```python
from build123d import *

# Parameters (mm, degrees)
F1_DEPTH = 15
F2_W     = 8.1
F2_H     = 8.1
F3_DEPTH = 15.001


with BuildPart() as f1:
    # F0 (on Top) → F1 (new body)
    with BuildSketch(Plane.XY):
        Polygon((9.68382, -9.550715), (10.192379, -9.560642), (10.750372, -9.002649), (11.202993, -8.356238), (11.104907, -7.857129), (10.443332, -6.402182), (9.825447, -5.605176), (9.499566, -5.342395), (8.382424, -4.808387), (7.960216, -4.101107), (8.739034, -1.961321), (9.517096, -1.690903), (10.716129, -1.999914), (11.134681, -2.008084), (12.120314, -1.794712), (13.562332, -1.105409), (13.958292, -0.786118), (14.027068, 0), (13.958292, 0.786118), (13.562332, 1.105409), (12.120314, 1.794712), (11.134681, 2.008084), (10.716129, 1.999914), (9.517096, 1.690903), (8.739034, 1.961321), (7.960216, 4.101107), (8.382424, 4.808387), (9.499566, 5.342395), (9.825447, 5.605176), (10.443332, 6.402182), (11.104907, 7.857129), (11.202993, 8.356238), (10.750372, 9.002649), (10.192379, 9.560642), (9.68382, 9.550715), (8.136095, 9.15184), (7.243903, 8.68174), (6.928526, 8.406442), (6.208641, 7.399001), (5.43879, 7.106025), (3.466753, 8.244581), (3.335552, 9.05778), (3.848079, 10.184939), (3.928805, 10.595713), (3.889828, 11.603424), (3.461401, 13.14323), (3.215719, 13.588618), (2.453486, 13.792858), (1.667367, 13.861634), (1.28417, 13.527134), (0.354935, 12.22672), (-0.026349, 11.293113), (-0.090983, 10.879501), (0.005123, 9.645024), (-0.396296, 8.925741), (-2.638814, 8.530325), (-3.262033, 9.068937), (-3.593939, 10.261836), (-3.796139, 10.628398), (-4.473741, 11.375294), (-5.791704, 12.279467), (-6.266198, 12.462733), (-6.981384, 12.129236), (-7.627795, 11.676614), (-7.706329, 11.174057), (-7.582274, 9.580582), (-7.274243, 8.620313), (-7.057892, 8.261922), (-6.190763, 7.378034), (-6.035921, 6.569004), (-7.499621, 4.824634), (-8.323248, 4.836637), (-9.344283, 5.537106), (-9.734799, 5.687937), (-10.733969, 5.824539), (-12.324777, 5.670005), (-12.806062, 5.505396), (-13.139559, 4.790209), (-13.343798, 4.027977), (-13.080922, 3.592515), (-11.961624, 2.451584), (-11.10841, 1.913973), (-10.712305, 1.778497), (-9.479894, 1.658779), (-8.841244, 1.138556), (-8.841244, -1.138556), (-9.479894, -1.658779), (-10.712305, -1.778497), (-11.10841, -1.913973), (-11.961624, -2.451584), (-13.080922, -3.592515), (-13.343798, -4.027977), (-13.139559, -4.790209), (-12.806062, -5.505396), (-12.324777, -5.670005), (-10.733969, -5.824539), (-9.734799, -5.687937), (-9.344283, -5.537106), (-8.323248, -4.836637), (-7.499621, -4.824634), (-6.035921, -6.569004), (-6.190763, -7.378034), (-7.057892, -8.261922), (-7.274243, -8.620313), (-7.582274, -9.580582), (-7.706329, -11.174057), (-7.627795, -11.676614), (-6.981384, -12.129236), (-6.266198, -12.462733), (-5.791704, -12.279467), (-4.473741, -11.375294), (-3.796139, -10.628398), (-3.593939, -10.261836), (-3.262033, -9.068937), (-2.638814, -8.530325), (-0.396296, -8.925741), (0.005123, -9.645024), (-0.090983, -10.879501), (-0.026349, -11.293113), (0.354935, -12.22672), (1.28417, -13.527134), (1.667367, -13.861634), (2.453486, -13.792858), (3.215719, -13.588618), (3.461401, -13.14323), (3.889828, -11.603424), (3.928805, -10.595713), (3.848079, -10.184939), (3.335552, -9.05778), (3.466753, -8.244581), (5.43879, -7.106025), (6.208641, -7.399001), (6.928526, -8.406442), (7.243903, -8.68174), (8.136095, -9.15184), align=None)
    extrude(amount=F1_DEPTH)

    # F2 (on face) → F3 (cut, through all)
    with BuildSketch(Plane.XY.offset(15)):
        Rectangle(F2_W, F2_H)
    extrude(amount=-F3_DEPTH, mode=Mode.SUBTRACT)


solid = f1.part
```
Check sheet for the modelled part. Datum: model origin and axes. Units: mm. A direction names the side the tool comes from. Coordinates: 2 decimals unless noted, no trailing zeros. Order: outer loops, then holes, each group sorted by start corner. A loop starts at its lowest first (then second) coordinate and runs counter-clockwise, first axis right, second up. Notation, with made-up numbers: M 22.5,-8 L 26.5,-8 A25 cw 26.5,9 Z; hole C 13,-35.75 d9. An arc over 180 degrees is marked long. Write each question's results on one line, items separated by ' | '. Start each with the question number.
1. Mould release check, pull along Y, two halves, no side actions. Record for faces 6 (the face through (0, -6, 0)), 7 (the face through (-12.5, -3, 7.4)), 8 (the face through (-8.827, 5.182, 7.395)): +Y half, -Y half, draft (parallel to the pull), parting line (faces both ways), or undercut.
2. Material ranges on probe 1 along Y at (x, z) = (9.75, 6); probe 2 along Y at (x, z) = (-7, 9.25); probe 3 along Y at (x, z) = (-1.75, 11.5), recorded low to high.
3. Go/stop test with flat-tipped pins: P1, Ø2.5, axis at y = 1.5, z = 8, coming from the +X side; P2, Ø8, axis at x = 6, z = 12, coming from the +Y side; P3, Ø2.5, axis at y = 2, z = 6, coming from the -X side. Record where each tip stops, or that it passes through.
4. Cross-section at A-A on x = -1. Record the cut outline in (y, z), and give its area (3 significant figures).
5. Access from +Z, -Z, +X, -X, +Y, -Y to the whole of each face (thin tool, end or side, straight path). Record for faces 1 (the face through (8.93, 5.07, 7.4)), 2 (the face through (-11.541, -5.746, 7.395)), 3 (the face through (6.574, 7.91, 7.395)), 4 (the face through (-7.645, 10.388, 7.395)), 5 (the face through (0, -4.05, 8)).
Checks:
1) face 6: draft | face 7: undercut | face 8: +Y half
2) probe 1: y = -9.55 to -5.54, -1.75 to 1.75, 5.54 to 9.55 | probe 2: y = -12.12 to -8.2, -5.42 to 5.42, 8.2 to 12.12 | probe 3: y = -8.69 to -4.05, 4.05 to 8.69
3) P1: stops at x = 14.01 | P2: stops at y = 13.83 | P3: stops at x = -12.74
4) outline: M -8.82,0 L -4.05,0 L -4.05,15 L -8.82,15 Z; M 4.05,0 L 8.82,0 L 8.82,15 L 4.05,15 Z | area: 143 mm²
5) face 1: +Z, -Z, +X | face 2: +Z, -Z, -X, -Y | face 3: +Z, -Z, +Y | face 4: +Z, -Z, -X | face 5: +Z, -Z
